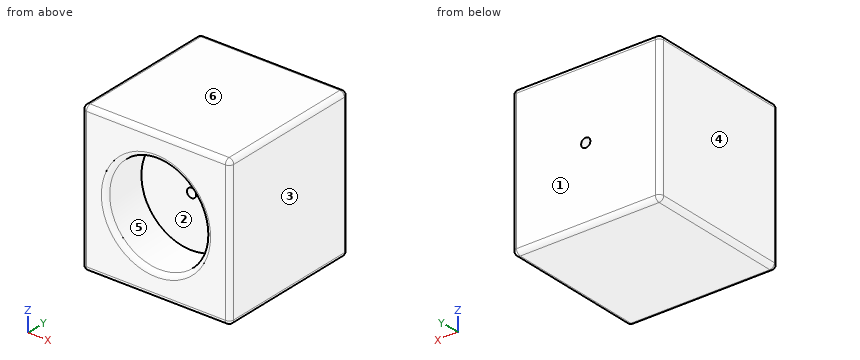
Autodesk Inventor part; units mm, degrees
ref_plane "YZ Plane" through (0, 0, 0) normal (1, 0, 0) x (0, 1, 0)
ref_plane "XZ Plane" through (0, 0, 0) normal (0, 1, 0) x (-1, 0, 0)
ref_plane "XY Plane" through (0, 0, 0) normal (0, 0, 1) x (1, 0, 0)
ref_plane "Work Plane3" through (101.6, 2.54, 38.1) normal (1, 0, 0) x (0, 0, -1)
sketch "Sketch1" plane through (101.6, 2.54, 38.1) normal (1, 0, 0) x (0, 0, -1)
  line L0 (88.9, -2.54) -> (-12.7, -2.54)
  line L1 (-12.7, -2.54) -> (-12.7, 99.06)
  line L2 (-12.7, 99.06) -> (88.9, 99.06)
  line L3 (88.9, 99.06) -> (88.9, -2.54)
  point P0 (38.1, -2.54)
extrude "Extrusion1" add sketch "Sketch1" along normal blind 101.6
sketch "Sketch2" plane through (101.6, 0, -50.8) normal (0, -1, 0) x (1, 0, 0)
  circle A0 centre (50.8, 50.8) radius 34.29
  point P0 (-101.6, 50.8)
  dimension "d3" = 68.58
extrude "Extrusion2" cut sketch "Sketch2" against normal blind 30.48
fillet "Fillet5" radius 3.175 13 edges at (152.4, 0, -50.8) (152.4, 101.6, -50.8) (101.6, 50.8, -50.8) (203.2, 50.8, -50.8) (152.4, 0, 50.8) (101.6, 0, 0) (203.2, 0, 0) (118.11, 0, 0) (152.4, 101.6, 50.8) (101.6, 101.6, 0) (203.2, 101.6, 0) (101.6, 50.8, 50.8) (203.2, 50.8, 50.8)
sketch "Sketch7" plane through (152.4, 30.48, 0) normal (0, -1, 0) x (1, 0, 0)
  point P0 (-152.4, 0)
  point P1 (0.1544, 0.9264)
hole "Hole1" at (152.5544, 30.48, 0.9264) direction (0, 1, 0) diameter 6.35 end through all
properties part number "1x2 Block v2"
The listing builds one solid part. Answer for the finished solid, in the listing's coordinates (mm). Face numbers are marked on the shaded views. A direction names the side the tool comes from. Round coordinates to 2 decimals unless told otherwise and drop trailing zeros. Write each loop counter-clockwise with the first axis right and the second up, starting at its lowest first coordinate (ties: lowest second). Pieces come first, ordered by that corner, then holes. Notation, with made-up numbers: M 81,9.25 L 108,9.25 A27 ccw 108,41.25 Z; hole C -6.5,-6 d9. An arc over 180 degrees is marked long. Write each question's results on one line, items separated by ' | '. Start each with the question number.
Item 1: A cutting plane is placed at A-A on y = 18.5. Write down the section's boundary in (x, z) (3 decimals).
Item 2: A cutting plane is placed at B-B on z = 0. Write down the section's boundary in (x, y) (3 decimals).
Item 3: Straight lines are drawn through the part: L1, parallel to Z at x = 152, y = 24; L2, parallel to Y at x = 149, z = 8; L3, parallel to Z at x = 122, y = 28.5. For each, find the intervals that lie inside material, in ascending order. Write a range as [from, to].
Item 4: A flat-ended cylindrical pin translates along its axis: pin 1 Ø6 at (x, z) = (168, 21.5) entering from -Y. Find the tip coordinate at first contact, or state that the pin passes through.
Item 5: For the marked faces 5 and 6, determine the directions among +Z, -Z, +X, -X, +Y, -Y from which every point of the face is accessible in a straight line to the end or side of a thin tool.
Item 6: For a pull along X with two mould halves and no side action, classify the marked faces 1, 2, 3 and 4 as pulls with the +X half, pulls with the -X half, needs draft (parallel to the pull), parting line crosses it, or undercut.
Check sheet entries:
1) outline: M 101.6,-47.625 A3.175 ccw 104.775,-50.8 L 200.025,-50.8 A3.175 ccw 203.2,-47.625 L 203.2,47.625 A3.175 ccw 200.025,50.8 L 104.775,50.8 A3.175 ccw 101.6,47.625 Z; hole C 152.4,0 d68.58
2) outline: M 101.6,3.175 A3.175 ccw 104.775,0 L 114.935,0 A3.175 ccw 118.11,3.175 L 118.11,30.48 L 149.518,30.48 L 149.518,101.6 L 104.775,101.6 A3.175 ccw 101.6,98.425 Z; M 155.591,30.48 L 186.69,30.48 L 186.69,3.175 A3.175 ccw 189.865,0 L 200.025,0 A3.175 ccw 203.2,3.175 L 203.2,98.425 A3.175 ccw 200.025,101.6 L 155.591,101.6 Z
3) L1: [-50.8, -34.29], [34.29, 50.8] | L2: [30.48, 101.6] | L3: [-50.8, -15.86], [15.86, 50.8]
4) pin 1: y = 30.48
5) face 5: -Y | face 6: +Z, +X, -X, +Y, -Y
6) face 1: needs draft | face 2: undercut | face 3: pulls with the +X half | face 4: pulls with the -X half
